Here's how the part is built. I have some questions about the finished solid (model axes, mm). Face numbers are marked on the shaded views. A direction names the side the tool comes from. Coordinates: 2 decimals unless noted, no trailing zeros. Loops run counter-clockwise (first coordinate to the right, second up) from the corner with the lowest first, then second, coordinate; pieces in that order, holes last. Notation, with made-up numbers: M 10.25,7 L 24.25,7 A24 cw 24.25,32 Z; hole C 27,-0.75 d7. An arc over 180 degrees is marked long. Use CSV: the item, a comma, the result in double quotes. Start each with the question number.
Q1. If we mould it in two halves opening along X, with no side actions, what happens to the marked faces 3, 4 and 5? For each: +X half, -X half, draft (parallel to the pull), parting line (faces both ways), or undercut.
Q2. Please list where these lines run through material, in increasing order: probe 1 along X at (y, z) = (7.5, 0); probe 2 along X at (y, z) = (4.75, 0); probe 3 along Y at (x, z) = (-14, -7.5). Write a range as [from, to].
Q3. If we section it at C-C (y = 3.5): Please give me the cut outline in (x, z), and give its area (3 significant figures).
Q4. If we section it at B-B (z = 0): Please give me the cut outline in (x, y).
Q5. Which directions (+Z, -Z, +X, -X, +Y, -Y) give clear straight access to the entire face, cutting with the end or side of a thin tool? Please do the marked faces 1 and 2.
Q6. For pin 1 Ø5 at (x, z) = (8, -11) entering from +Y; pin 2 Ø1.5 at (y, z) = (11.5, -4) entering from +X; pin 3 Ø3 at (x, z) = (0, -6) entering from +Y, each with a flat end and sliding along its axis, tell me the tip position at first contact or that it passes through.
Q7. If we section it at A-A (x = 0): State how many separate pieces and enclosed holes the cut face has, and give its area (3 significant figures).
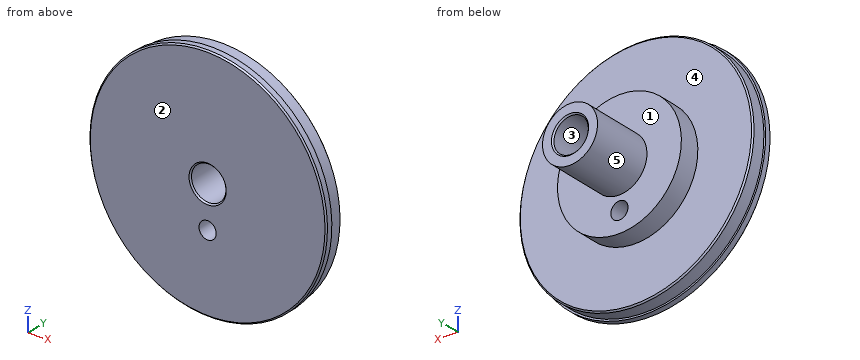
from build123d import *

# Parameters (mm, degrees)
SKETCH1_R           = 17.25
BOSS_EXTRUDE1_DEPTH = 15
SKETCH2_OUTSIDE_W   = 46.708
SKETCH2_OUTSIDE_H   = 46.708
SKETCH2_OUTSIDE_R   = 17
CUT_EXTRUDE1_DEPTH  = 14
SKETCH3_OUTSIDE_W   = 46.708
SKETCH3_OUTSIDE_H   = 46.708
SKETCH3_OUTSIDE_R   = 9
CUT_EXTRUDE4_DEPTH  = 12
SKETCH6_OUTSIDE_W   = 46.708
SKETCH6_OUTSIDE_H   = 46.708
SKETCH6_OUTSIDE_R   = 4
CUT_EXTRUDE5_DEPTH  = 9
SKETCH7_R           = 2.5
CUT_EXTRUDE6_DEPTH  = 29.637824638
SKETCH8_R           = 1.25
CUT_EXTRUDE7_DEPTH  = 27.002403735
CHAMFER1_SIZE       = 0.2


with BuildPart() as part:
    # Sketch1 → Boss-Extrude1 (new body)
    with BuildSketch(Plane(origin=(0, 0, 0), x_dir=(1, 0, 0), z_dir=(0, 1, 0))):
        with Locations(Location((0, 0, 0), (0, 0, 270))):
            Circle(SKETCH1_R)
    extrude(amount=BOSS_EXTRUDE1_DEPTH)

    # Sketch2 outside → Cut-Extrude1 (cut)
    with BuildSketch(Plane(origin=(0, 15, 0), x_dir=(1, 0, 0), z_dir=(0, 1, 0))):
        Rectangle(SKETCH2_OUTSIDE_W, SKETCH2_OUTSIDE_H)
        with Locations(Location((0, 0, 0), (0, 0, 270))):
            Circle(SKETCH2_OUTSIDE_R, mode=Mode.SUBTRACT)
    extrude(amount=-CUT_EXTRUDE1_DEPTH, mode=Mode.SUBTRACT)

    # Sketch3 outside → Cut-Extrude4 (cut)
    with BuildSketch(Plane(origin=(0, 15, 0), x_dir=(1, 0, 0), z_dir=(0, 1, 0))):
        Rectangle(SKETCH3_OUTSIDE_W, SKETCH3_OUTSIDE_H)
        with Locations(Location((0, 0, 0), (0, 0, 270))):
            Circle(SKETCH3_OUTSIDE_R, mode=Mode.SUBTRACT)
    extrude(amount=-CUT_EXTRUDE4_DEPTH, mode=Mode.SUBTRACT)

    # Sketch6 outside → Cut-Extrude5 (cut)
    with BuildSketch(Plane(origin=(0, 15, 0), x_dir=(1, 0, 0), z_dir=(0, 1, 0))):
        Rectangle(SKETCH6_OUTSIDE_W, SKETCH6_OUTSIDE_H)
        with Locations(Location((0, 0, 0), (0, 0, 270))):
            Circle(SKETCH6_OUTSIDE_R, mode=Mode.SUBTRACT)
    extrude(amount=-CUT_EXTRUDE5_DEPTH, mode=Mode.SUBTRACT)

    # Sketch7 → Cut-Extrude6 (cut, through all)
    with BuildSketch(Plane(origin=(0, 15, 0), x_dir=(1, 0, 0), z_dir=(0, 1, 0))):
        with Locations(Location((0, 0, 0), (0, 0, 270))):
            Circle(SKETCH7_R)
    extrude(amount=-CUT_EXTRUDE6_DEPTH, mode=Mode.SUBTRACT)

    # Sketch8 → Cut-Extrude7 (cut, through all)
    with BuildSketch(Plane(origin=(0, 6, 0), x_dir=(1, 0, 0), z_dir=(0, 1, 0))):
        with Locations(Location((0, 6, 0), (0, 0, 270))):
            Circle(SKETCH8_R)
    extrude(amount=-CUT_EXTRUDE7_DEPTH, mode=Mode.SUBTRACT)

    # Chamfer1
    chamfer1_edges = [part.edges().sort_by_distance(p)[0] for p in [
        (0, 0, -17.25),
        (0, 3, -17),
        (0, 0, -2.5),
        (0, 15, -2.5),
    ]]
    chamfer(chamfer1_edges, length=CHAMFER1_SIZE)


solid = part.part
Results below:
1,face 3,"undercut"
1,face 4,"draft"
1,face 5,"parting line"
2,probe 1,"[-4, -2.5], [2.5, 4]"
2,probe 2,"[-9, -2.5], [2.5, 9]"
2,probe 3,"[0, 3]"
3,outline,"C 0,0 d18; hole C 0,0 d5; hole C 0,-6 d2.5"
3,area,"230 mm^2"
4,outline,"M -17.25,0.2 L -17.05,0 L -2.7,0 L -2.5,0.2 L -2.5,14.8 L -2.7,15 L -4,15 L -4,6 L -9,6 L -9,3 L -16.8,3 L -17,2.8 L -17,1 L -17.25,1 Z; M 2.5,0.2 L 2.7,0 L 17.05,0 L 17.25,0.2 L 17.25,1 L 17,1 L 17,2.8 L 16.8,3 L 9,3 L 9,6 L 4,6 L 4,15 L 2.7,15 L 2.5,14.8 Z"
5,face 1,"+Y"
5,face 2,"+Z, -Z, +X, -X, -Y"
6,pin 1,"y = 3"
6,pin 2,"x = 2.33"
6,pin 3,"y = 6"
7,separate pieces,"3"
7,enclosed holes,"0"
7,area,"138 mm^2"
